Part model, mm, in its own coordinate system. A direction names the side the tool comes from. Coordinates: 2 decimals unless noted, no trailing zeros. Order: outer loops, then holes, each group sorted by start corner. A loop starts at its lowest first (then second) coordinate and runs counter-clockwise, first axis right, second up. Notation, with made-up numbers: M -22.5,54.5 L -17.5,54.5 A24 cw -17.5,72.5 Z; hole C 47.25,-16.75 d6. An arc over 180 degrees is marked long. Write item = value, one per line. Start each with the question number.
Autodesk Inventor part; units mm, degrees
ref_plane "YZ Plane" through (0, 0, 0) normal (1, 0, 0) x (0, 1, 0)
ref_plane "XZ Plane" through (0, 0, 0) normal (0, 1, 0) x (-1, 0, 0)
ref_plane "XY Plane" through (0, 0, 0) normal (0, 0, 1) x (1, 0, 0)
sketch "Эскиз1" plane through (0, 0, 0) normal (0, 0, 1) x (1, 0, 0)
  line L0 (0, 0) -> (0, 8)
  line L1 (0, 8) -> (0, 16)
  line L2 (0, 0) -> (0, 20)
  line L3 (0, 20) -> (-75, 20)
  line L4 (-75, 20) -> (-75, 0)
  line L5 (-75, 0) -> (-51, 0)
  line L6 (-51, 0) -> (-51, 8)
  line L7 (-51, 8) -> (-34, 8)
  line L8 (-34, 8) -> (-34, 20)
  line L9 (0, 20) -> (-49, 20)
  line L10 (-49, 20) -> (-49, 20)
  circle A0 centre (-49, 20) radius 2
  point P0 (-47, 20)
  point P1 (-51, 20)
  dimension "d22" = 20
  dimension "d23" = 75
  dimension "d26" = 24
  dimension "d27" = 8
  dimension "d28" = 17
  dimension "d29" = 49
  dimension "d30" = 0
  dimension "d31" = 4
revolve "Вращение1" add sketch "Эскиз1" angle 360 about axis through (0, 8, 0) along (0, 1, 0) contours L8 L7 L6 L5 L4 L3 A0
sketch "Эскиз2" plane through (0, 20, 0) normal (0, 1, 0) x (1, 0, 0)
  line L0 (0, 0) -> (41.7812, 49.7929)
  line L1 (0, 0) -> (65, 0) construction
  line L2 (0, 0) -> (-32.5, 56.2917)
  line L3 (0, 0) -> (65, 0) construction
  line L4 (0, 0) -> (-11.2871, -64.0125)
  line L5 (0, 0) -> (65, 0) construction
  circle A0 centre (-32.5, 56.2917) radius 1.5
  circle A1 centre (41.7812, 49.7929) radius 1.5
  circle A2 centre (-11.2871, -64.0125) radius 1.5
  dimension "d11" = 65
  dimension "d12" = 50
  dimension "d13" = 65
  dimension "d14" = 120
  dimension "d15" = 65
  dimension "d16" = 100
  dimension "d17" = 3
  dimension "d18" = 3
  dimension "d19" = 3
extrude "Выдавливание1" cut sketch "Эскиз2" against normal through all
sketch "Эскиз3" plane through (0, 0, 0) normal (0, -1, 0) x (1, 0, 0)
  circle A0 centre (0, 0) radius 53
  circle A1 centre (0, 0) radius 55
  dimension "d32" = 106
  dimension "d33" = 110
extrude "Выдавливание2" cut sketch "Эскиз3" against normal blind 1.5
properties part number "Корпус дросселя" material "Чугун, серый"
Item 1: Cut at C-C, the plane y = 14.5. Write the cut outline in (x, z).
Item 2: Cut at D-D, the plane x = -59.5. Write the cut outline in (y, z).
Item 3: Cut at A-A, the plane x = 0. Write the cut outline in (y, z), and give its area (3 significant figures).
Item 4: 3-axis set-ups, long thin cutter, end or side, ignore diameter. For faces 1 (the cylindrical face through (11.056, 4.056, -49.787)), 2 (the cylindrical face through (-18.28, 14.08, 28.67)): which of +Z, -Z, +X, -X, +Y, -Y reach the whole face in a straight line?
Item 5: Flat gauge pins, fed straight in: pin 1 (12 mm diameter, centred on x = -41, y = 7.5, fed in from +Z); pin 2 (8 mm diameter, centred on x = -17, z = -23, fed in from +Y); pin 3 (12 mm diameter, centred on x = -37.5, y = 18, fed in from -Z); pin 4 (1.5 mm diameter, centred on y = 3, z = -32, fed in from +X). Where does each tip first touch, or does it go through?
Item 6: Cut at B-B, the plane z = 0. Write the cut outline in (x, y).
Item 7: Pull direction X, two halves, no side cores. Call faces 3 (the flat face through (28, 0, 43)), 4 (the flat face through (-33, 8, -11)), 5 (the cylindrical face through (9.764, 9.86, -74.362)): pulls with the +X half, pulls with the -X half, needs draft (parallel to the pull), parting line crosses it, or undercut.
Item 8: Wall check: line 1 along Z through (x, y) = (3.5, 1); line 2 along Z through (x, y) = (-32.5, 6); line 3 along Z through (x, y) = (-40, 7). Give the ranges that are in metal, low to high. Write a range as [from, to].
Filled sheet:
q1.outline = C 0,0 d150; hole C -32.5,-56.29 d3; hole C 0,0 d68; hole C -11.29,64.01 d3; hole C 41.78,-49.79 d3
q2.outline = M 0,-45.66 L 20,-45.66 L 20,45.66 L 0,45.66 Z
q3.outline = M 0,-75 L 20,-75 L 20,-51 A2 cw 20,-47 L 20,-34 L 8,-34 L 8,-51 L 0,-51 L 0,-53 L 1.5,-53 L 1.5,-55 L 0,-55 Z; M 0,51 L 8,51 L 8,34 L 20,34 L 20,47 A2 cw 20,51 L 20,75 L 0,75 L 0,55 L 1.5,55 L 1.5,53 L 0,53 Z
q3.area = 1,350 mm2
q4.face_1 = -Y
q4.face_2 = +Y, -Y
q5.pin_1 = 66.33
q5.pin_2 = through
q5.pin_3 = -68.06
q5.pin_4 = 68.18
q6.outline = M -75,0 L -55,0 L -55,1.5 L -53,1.5 L -53,0 L -51,0 L -51,8 L -34,8 L -34,20 L -47,20 A2 cw -51,20 L -75,20 Z; M 34,8 L 51,8 L 51,0 L 53,0 L 53,1.5 L 55,1.5 L 55,0 L 75,0 L 75,20 L 51,20 A2 cw 47,20 L 34,20 Z
q7.face_3 = needs draft
q7.face_4 = undercut
q7.face_5 = parting line crosses it
q8.line_1 = [-74.92, -54.89], [-52.88, -50.88], [50.88, 52.88], [54.89, 74.92]
q8.line_2 = [-67.59, -57.79], [-54.79, -39.3], [39.3, 67.59]
q8.line_3 = [-63.44, -31.64], [31.64, 63.44]
